The drawing under review shows one solid part. Ordinate dimensions are in mm from its lowest x, y, z. A direction names the side the tool comes from. Coordinates: 2 decimals unless noted, no trailing zeros. Write each loop counter-clockwise with the first axis right and the second up, starting at its lowest first coordinate (ties: lowest second). Pieces come first, ordered by that corner, then holes.
1) For line 1 (Y direction, x = 6.25, z = 9.5); line 2 (X direction, y = 0.5, z = 6); line 3 (X direction, y = 15.25, z = 1), list the stretches that pass through material, from the lowest coordinate up.
2) For P1, Ø1, axis at x = 3, y = 11, coming from the -Z side; P2, Ø3, axis at x = 3.5, y = 14, coming from the -Z side; P3, Ø5, axis at y = 2, z = 8.5, coming from the +X side; P4, Ø3, axis at y = 5, z = 3, coming from the -X side, all flat-tipped, find the tip position at first contact; note any pin that passes through.
3) Add section A-A, the plane z = 6. State the section outline as (x, y) points, then the cut area to 3 significant figures.
4) Machinability: for the marked faces 1 and 2, which of the approach directions +Z, -Z, +X, -X, +Y, -Y give a long, thin tool a straight path to every point of the face, cutting with its end or side? Answer none if there is none.
5) Add section C-C, the plane y = 14.75. State the section outline as (x, z) points, then the cut area to 3 significant figures.
6) Add section D-D, the plane y = 10.5. State the section outline as (x, z) points.
7) Add section B-B, the plane x = 5. State the section outline as (y, z) points.
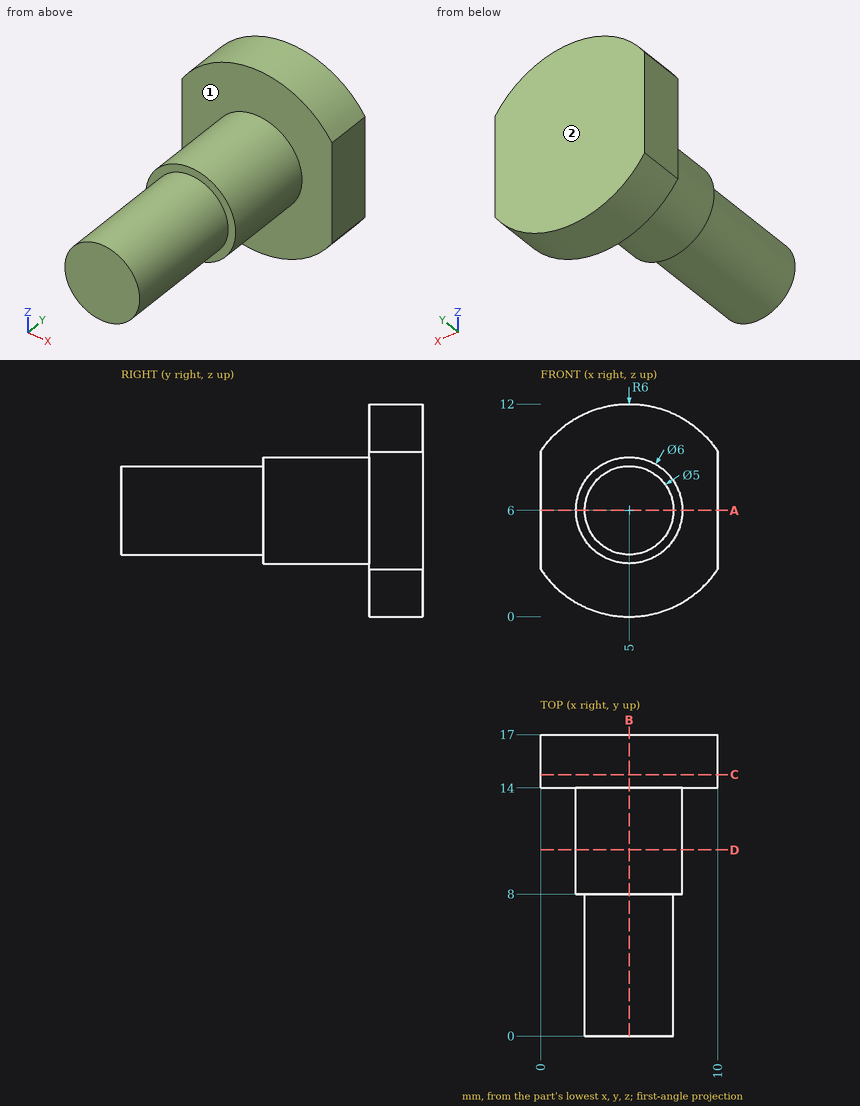
Geometry results:
1. line 1: y = 14 to 17
1. line 2: x = 2.5 to 7.5
1. line 3: x = 1.68 to 8.32
2. P1: stops at z = 3.4
2. P2: stops at z = 0
2. P3: stops at x = 7.5
2. P4: stops at x = 3
3. outline: (0, 14) - (2, 14) - (2, 8) - (2.5, 8) - (2.5, 0) - (7.5, 0) - (7.5, 8) - (8, 8) - (8, 14) - (10, 14) - (10, 17) - (0, 17) - close
3. area: 106 mm2
4. face 1: -Y
4. face 2: +Z, -Z, +X, -X, +Y
5. outline: (0, 2.68) arc R6 ccw to (10, 2.68) - (10, 9.32) arc R6 ccw to (0, 9.32) - close
5. area: 104 mm2
6. outline: circle Ø6 at (5, 6)
7. outline: (0, 3.5) - (8, 3.5) - (8, 3) - (14, 3) - (14, 0) - (17, 0) - (17, 12) - (14, 12) - (14, 9) - (8, 9) - (8, 8.5) - (0, 8.5) - close
